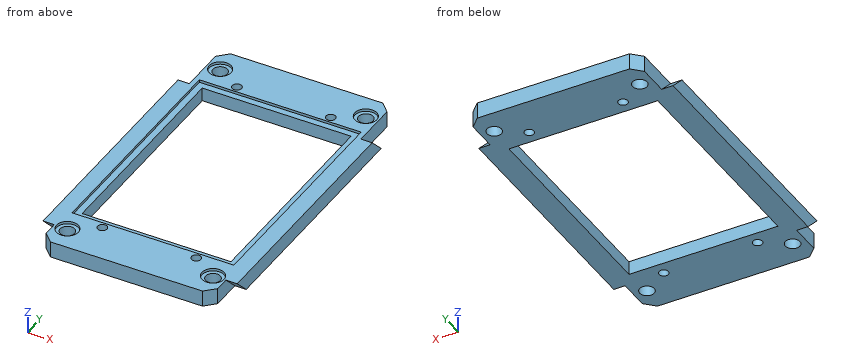
Autodesk Inventor part; units mm, degrees
ref_plane "YZ Plane" through (0, 0, 0) normal (1, 0, 0) x (0, 1, 0)
ref_plane "XZ Plane" through (0, 0, 0) normal (0, 1, 0) x (-1, 0, 0)
ref_plane "XY Plane" through (0, 0, 0) normal (0, 0, 1) x (1, 0, 0)
sketch "Szkic1" plane through (0, 0, 0) normal (0, 0, 1) x (1, 0, 0)
  circle A0 centre (-15, -14.1421) radius 2
  circle A1 centre (-60, -14.1421) radius 2
  circle A2 centre (-15, -98.9949) radius 2
  circle A3 centre (-60, -98.9949) radius 2
  line L0 (-75, -84.8528) -> (0, -84.8528) construction
  line L1 (-75, -27.2843) -> (0, -27.2843) construction
  line L2 (-12.5, -21.2132) -> (-62.5, -21.2132) construction
  line L3 (-62.5, -21.2132) -> (-62.5, -91.9239) construction
  line L4 (-62.5, -91.9239) -> (-12.5, -91.9239) construction
  line L5 (-12.5, -91.9239) -> (-12.5, -21.2132) construction
  line L6 (-15, -98.9949) -> (-60, -14.1421) construction
  line L7 (-15, -14.1421) -> (-60, -98.9949) construction
  line L8 (-7.5, -6.5685) -> (-67.5, -6.5685)
  line L9 (-67.5, -6.5685) -> (-67.5, -106.5685)
  line L10 (-67.5, -106.5685) -> (-7.5, -106.5685)
  line L11 (-7.5, -106.5685) -> (-7.5, -6.5685)
  circle A4 centre (-15, -14.1421) radius 2.25
  circle A5 centre (-60, -14.1421) radius 2.25
  circle A6 centre (-60, -98.9949) radius 2.25
  circle A7 centre (-15, -98.9949) radius 2.25
  line L12 (-12.5, -21.2132) -> (-62.5, -21.2132)
  line L13 (-62.5, -21.2132) -> (-62.5, -91.9239)
  line L14 (-62.5, -91.9239) -> (-12.5, -91.9239)
  line L15 (-12.5, -91.9239) -> (-12.5, -21.2132)
  line L16 (-14.5, -23.2132) -> (-60.5, -23.2132)
  line L17 (-60.5, -23.2132) -> (-60.5, -89.9239)
  line L18 (-60.5, -89.9239) -> (-14.5, -89.9239)
  line L19 (-14.5, -89.9239) -> (-14.5, -23.2132)
  ellipse E0 centre (-7.5, -14.1421) end of major axis (-7.5, -18.3848) minor radius 3
  ellipse E1 centre (-67.5, -14.1421) end of major axis (-67.5, -18.3848) minor radius 3
  ellipse E2 centre (-67.5, -98.9949) end of major axis (-67.5, -103.2376) minor radius 3
  ellipse E3 centre (-7.5, -98.9949) end of major axis (-7.5, -103.2376) minor radius 3
  line L20 (-11.5, -94.4949) -> (-11.5, -106.5685)
  line L21 (-11.5, -94.4949) -> (-7.5, -94.4949)
  line L22 (-37.5, -106.5685) -> (-37.5, -6.5685) construction
  line L23 (-63.5, -94.4949) -> (-63.5, -106.5685)
  line L24 (-63.5, -94.4949) -> (-67.5, -94.4949)
  line L25 (-7.5, -56.5685) -> (-67.5, -56.5685) construction
  line L26 (-11.5, -18.6421) -> (-11.5, -6.5685)
  line L27 (-11.5, -18.6421) -> (-7.5, -18.6421)
  line L28 (-63.5, -18.6421) -> (-63.5, -6.5685)
  line L29 (-63.5, -18.6421) -> (-67.5, -18.6421)
  point P0 (0, 0)
  point P1 (-37.5, -56.5685)
  point P2 (-37.5, -91.9239)
  point P3 (-12.5, -56.5685)
  point P4 (-37.5, -56.5685)
  dimension "d0" = 50
  dimension "d1" = 70.7107
  dimension "d2" = 4.5
  dimension "d3" = 2
  dimension "d4" = 60
  dimension "d5" = 100
  dimension "d15" = 4
  dimension "d16" = 4.5
extrude "Wyciągnięcie proste1" add sketch "Szkic1" along normal blind 5 contours L11 E0 L27 L26 L8 | L26 L27 L11 L21 L20 L10 L23 L24 L9 L29 L28 L8 | L11 E0 | L28 L29 L9 E1 L8 | E1 L9 | L11 E3 L10 L20 L21 | L24 L23 L10 L9 E2 | L11 E3 | E2 L9 | L15 L14 L13 L12 picked at (-8.4985, -14.0649) picked at (-66.5015, -14.2193) picked at (-8.4985, -98.9177) picked at (-66.5015, -99.0721)
sketch "Szkic2" plane through (0, 0, 5) normal (0, 0, 1) x (1, 0, 0)
  line L0 (-62.5, -21.2132) -> (-62.5, -91.9239)
  line L1 (-12.5, -21.2132) -> (-62.5, -21.2132) construction
  line L2 (-12.5, -91.9239) -> (-12.5, -21.2132)
  line L3 (-62.5, -91.9239) -> (-12.5, -91.9239) construction
  line L4 (-12.5, -21.2132) -> (-62.5, -21.2132)
  line L5 (-62.5, -21.2132) -> (-62.5, -91.9239)
  line L6 (-62.5, -91.9239) -> (-12.5, -91.9239)
  line L7 (-12.5, -91.9239) -> (-12.5, -21.2132)
  circle A0 centre (-15, -14.1421) radius 3.4
  circle A1 centre (-60, -14.1421) radius 3.4
  circle A2 centre (-60, -98.9949) radius 3.4
  circle A3 centre (-15, -98.9949) radius 3.4
  point P0 (0, 0)
  dimension "d10" = 6.8
  dimension "d11" = 6.8
extrude "Wyciągnięcie proste2" cut sketch "Szkic2" against normal blind 0.8
chamfer "Faza1" distance 3 angle 45 4 edges at (-7.5, -106.5685, 2.5) (-67.5, -106.5685, 2.5) (-67.5, -6.5685, 2.5) (-7.5, -6.5685, 2.5)
sketch "Szkic3" plane through (0, 0, 5) normal (0, 0, 1) x (1, 0, 0)
  point P0 (0, 0)
ref_plane "Płaszczyzna konstrukcyjna1" through (-7.5, -6.5685, 0) normal (0, 0.7071, -0.7071) x (-1, 0, 0)
sketch "Szkic4" plane through (-7.5, -6.5685, 0) normal (0, 0.7071, -0.7071) x (-1, 0, 0)
  circle A0 centre (0, -65.3553) radius 3
  circle A1 centre (0, -5.3553) radius 3
  circle A2 centre (60, -65.3553) radius 3
  circle A3 centre (60, -5.3553) radius 3
  line L0 (0, -68.5894) -> (0, -2.1213)
  line L1 (57, -70.7107) -> (3, -70.7107)
  line L2 (3, 3.5355) -> (57, 3.5355)
  line L3 (0, -76.8553) -> (3.5, -76.8553)
  line L4 (3.5, -76.8553) -> (3.5, -61.8553)
  line L5 (3.5, -61.8553) -> (0, -61.8553)
  line L6 (0, -61.8553) -> (0, -76.8553)
  line L7 (0, -65.3553) -> (0, -5.3553) construction
  line L8 (0, -5.3553) -> (60, -5.3553) construction
  line L9 (0, -35.3553) -> (60, -35.3553) construction
  line L10 (60, -2.1213) -> (60, -68.5894) construction
  line L11 (30, -70.7107) -> (30, -5.3553) construction
  line L12 (0, 6.1447) -> (3.5, 6.1447)
  line L13 (3.5, 6.1447) -> (3.5, -8.8553)
  line L14 (3.5, -8.8553) -> (0, -8.8553)
  line L15 (0, -8.8553) -> (0, 6.1447)
  line L16 (60, -76.8553) -> (56.5, -76.8553)
  line L17 (56.5, -76.8553) -> (56.5, -61.8553)
  line L18 (56.5, -61.8553) -> (60, -61.8553)
  line L19 (60, -61.8553) -> (60, -76.8553)
  line L20 (56.5, 6.1447) -> (56.5, -8.8553)
  line L21 (60, 6.1447) -> (56.5, 6.1447)
  line L22 (60, -8.8553) -> (60, 6.1447)
  line L23 (56.5, -8.8553) -> (60, -8.8553)
  point P0 (-7.5, 4.6447)
  point P1 (56.5, -70.7107)
  point P2 (0, -8.3553)
  point P3 (0, -8.8553)
  point P4 (0, -2.1213)
  point P5 (0, -2.3553)
  point P6 (3.5, -70.7107)
  point P7 (0, -61.8553)
  point P8 (60, -68.3553)
  point P9 (60, -62.3553)
  point P10 (60, -8.3553)
  point P11 (60, -2.3553)
  point P12 (0, -62.3553)
  point P13 (0, -68.3553)
  dimension "d18" = 3.5
  dimension "d19" = 15
  dimension "d22" = 3.5
extrude "Wyciągnięcie proste3" cut sketch "Szkic4" against normal through all contours A0 L0 | A0 L0 L5 L4 L3 L6 | L20 L21 L22 A3 L23 | L0 A1 L15 L12 L13 L14 | L17 L18 L19 A2 L16 | L0 A1 | A1 L0 | A2 L19 | L22 A3 picked at (1.6278, -64.5387) picked at (59.5353, -64.4698) picked at (59.296, -4.4408)
chamfer "Faza2" distance 3 angle 45 4 edges at (-11, -6.5685, 2.5) (-64, -6.5685, 2.5) (-11, -106.5685, 2.5) (-64, -106.5685, 2.5)
sketch "Szkic5" plane through (0, 0, 5) normal (0, 0, 1) x (1, 0, 0)
  point P0 (0, 0)
sketch "Szkic6" plane through (0, 0, 5) normal (0, 0, 1) x (1, 0, 0)
  circle A0 centre (-52, -19.2132) radius 1.45
  line L0 (-14, -6.5685) -> (-61, -6.5685) construction
  line L1 (-37.5, -6.5685) -> (-37.5, -106.5685) construction
  line L2 (-61, -106.5685) -> (-14, -106.5685) construction
  line L3 (-67.5, -19.0919) -> (-67.5, -94.0452) construction
  line L4 (-67.5, -56.5685) -> (-7.5, -56.5685) construction
  line L5 (-7.5, -94.0452) -> (-7.5, -19.0919) construction
  line L6 (-62.5, -21.2132) -> (-12.5, -21.2132) construction
  line L7 (-64, -9.5685) -> (-64, -24.0919) construction
  circle A1 centre (-23, -19.2132) radius 1.45
  circle A2 centre (-52, -93.9239) radius 1.45
  circle A3 centre (-23, -93.9239) radius 1.45
  point P0 (0, 0)
  dimension "d26" = 2.9
  dimension "d27" = 2
  dimension "d28" = 12
extrude "Wyciągnięcie proste4" cut sketch "Szkic6" against normal through all
properties part number "mirror_bracket"
Build history of the part. All positions in model axes, mm. Coordinates: 2 decimals unless noted, no trailing zeros. Order: outer loops, then holes, each group sorted by start corner. A loop starts at its lowest first (then second) coordinate and runs counter-clockwise, first axis right, second up. Notation, with made-up numbers: (82.25, -36.75) - (137.25, -36.75) arc R27 ccw to (137.25, -13.75) - close; hole circle Ø2 at (64.5, 61). An arc over 180 degrees is marked (long way). Write item = value, one per line. Start each with the question number.
1) Wall check: line 1 along Y through (x, z) = (-60, 0.5); line 2 along Y through (x, z) = (-23, 3.25); line 3 along X through (y, z) = (-94, 3). Give the ranges that are in metal, low to high. Write a range as from..to.
2) Flat gauge pin, fed straight in: pin 1 Ø6 at (x, y) = (-60, -98.99) entering from -Z. Where does the tip first touch, or does it go through?
3) Saw through at B-B on y = -71. Write the cut outline in (x, z).
4) Saw through at A-A on x = -52. Write the cut outline in (y, z).
From the geometry:
q1.line_1 = -106.57..-101.24, -96.74..-89.92, -23.21..-16.39, -11.89..-6.57
q1.line_2 = -106.57..-95.37, -92.47..-89.92, -23.21..-20.66, -17.76..-6.57
q1.line_3 = -67.5..-53.45, -50.55..-24.45, -21.55..-7.5
q2.pin_1 = 0
q3.outline = (-67.5, 0) - (-60.5, 0) - (-60.5, 4.2) - (-62.5, 4.2) - (-62.5, 5) - (-67.5, 5) - close; (-14.5, 0) - (-7.5, 0) - (-7.5, 5) - (-12.5, 5) - (-12.5, 4.2) - (-14.5, 4.2) - close
q4.outline = (-106.57, 0) - (-95.37, 0) - (-95.37, 5) - (-106.57, 5) - close; (-92.47, 0) - (-89.92, 0) - (-89.92, 4.2) - (-91.92, 4.2) - (-91.92, 5) - (-92.47, 5) - close; (-23.21, 0) - (-20.66, 0) - (-20.66, 5) - (-21.21, 5) - (-21.21, 4.2) - (-23.21, 4.2) - close; (-17.76, 0) - (-6.57, 0) - (-6.57, 5) - (-17.76, 5) - close
